Geometry check sheet. Reference: the model listing, model coordinates, mm. A direction names the side the tool comes from. Coordinates: 2 decimals unless noted, no trailing zeros. Loops run counter-clockwise (first coordinate to the right, second up) from the corner with the lowest first, then second, coordinate; pieces in that order, holes last.
Autodesk Inventor part; units mm, degrees
ref_plane "YZ Plane" through (0, 0, 0) normal (1, 0, 0) x (0, 1, 0)
ref_plane "XZ Plane" through (0, 0, 0) normal (0, 1, 0) x (-1, 0, 0)
ref_plane "XY Plane" through (0, 0, 0) normal (0, 0, 1) x (1, 0, 0)
sketch "Sketch1" plane through (0, 0, 0) normal (0, 1, 0) x (-1, 0, 0)
  line L0 (0, 0) -> (60, 0)
  line L1 (60, 0) -> (60, -140)
  line L2 (60, -140) -> (0, -140)
  line L3 (0, -140) -> (0, 0)
  line L4 (30, -20.8594) -> (30, -183.1932) construction
  line L5 (42.5, -21.7206) -> (42.5, -191.0157) construction
  line L6 (17.5, -21.7206) -> (17.5, -184.1979) construction
  circle A0 centre (42.5, -21) radius 1.5
  circle A1 centre (42.5, -41) radius 1.5
  circle A2 centre (42.5, -99) radius 1.5
  circle A3 centre (42.5, -119) radius 1.5
  circle A4 centre (17.5, -99) radius 1.5
  circle A5 centre (17.5, -119) radius 1.5
  circle A6 centre (17.5, -41) radius 1.5
  circle A7 centre (17.5, -21) radius 1.5
  dimension "d0" = 140
  dimension "d1" = 60
  dimension "d2" = 30
  dimension "d3" = 12.5
  dimension "d4" = 12.5
  dimension "d5" = 3
  dimension "d6" = 3
  dimension "d7" = 3
  dimension "d8" = 3
  dimension "d9" = 3
  dimension "d10" = 3
  dimension "d11" = 3
  dimension "d12" = 3
  dimension "d13" = 20
  dimension "d14" = 20
  dimension "d15" = 20
  dimension "d16" = 20
  dimension "d17" = 21
  dimension "d18" = 21
  dimension "d19" = 21
  dimension "d20" = 21
extrude "Extrusion1" add sketch "Sketch1" along normal blind 5
sketch "Sketch2" plane through (0, 0, 0) normal (0, -1, 0) x (1, 0, 0)
  circle A0 centre (-52.5, -120) radius 2.5
  circle A1 centre (-52.5, -20) radius 2.5
  circle A2 centre (-7.5, -120) radius 2.5
  circle A3 centre (-7.5, -20) radius 2.5
  line L0 (-60, -140) -> (-60, 0)
  line L1 (0, -140) -> (-60, -140)
  line L2 (-60, 0) -> (0, 0)
  line L3 (0, 0) -> (0, -140)
  dimension "d23" = 5
  dimension "d24" = 5
  dimension "d25" = 5
  dimension "d26" = 5
  dimension "d27" = 7.5
  dimension "d28" = 20
  dimension "d29" = 7.5
  dimension "d30" = 20
  dimension "d31" = 20
  dimension "d32" = 7.5
  dimension "d33" = 20
  dimension "d34" = 7.5
extrude "Extrusion2" cut sketch "Sketch2" against normal blind 10 contours A0 | A1 | A2 | A3
sketch "Sketch3" plane through (0, 0, 0) normal (0, -1, 0) x (1, 0, 0)
  line L0 (-68.3542, -70) -> (15.9682, -70) construction
  line L1 (0, -140) -> (-60, -140)
  line L2 (-35, -136) -> (-25, -136)
  line L3 (-25, -136) -> (-25, -131)
  line L4 (-25, -131) -> (-35, -131)
  line L5 (-35, -131) -> (-35, -136)
  line L6 (-60, -140) -> (-60, 0)
  line L7 (-35, -4) -> (-25, -4)
  line L8 (-25, -4) -> (-25, -9)
  line L9 (-25, -9) -> (-35, -9)
  line L10 (-35, -9) -> (-35, -4)
  point P0 (0, 0)
  dimension "d40" = 70
  dimension "d41" = 10
  dimension "d42" = 25
  dimension "d43" = 4
  dimension "d44" = 5
extrude "Extrusion3" cut sketch "Sketch3" against normal blind 10
fillet "Fillet2" radius 5 4 edges at (0, 2.5, -140) (-60, 2.5, -140) (-60, 2.5, 0) (0, 2.5, 0)
sketch "Sketch4" plane through (0, 5, 0) normal (0, 1, 0) x (1, 0, 0)
  circle A0 centre (-10, 65.5) radius 1.5
  circle A1 centre (-30, 65.5) radius 1.5
  circle A2 centre (-50, 65.5) radius 1.5
  line L0 (3.8133, 65.5) -> (-51.9818, 65.5) construction
  line L1 (-55, 0) -> (-5, 0)
  line L2 (0, 5) -> (0, 135)
  point P0 (0, 0)
  dimension "d49" = 3
  dimension "d50" = 3
  dimension "d51" = 3
  dimension "d52" = 65.5
  dimension "d53" = 10
  dimension "d54" = 30
  dimension "d55" = 50
extrude "Extrusion4" cut sketch "Sketch4" against normal blind 10
fillet "Fillet3" radius 2 8 edges at (-25, 2.5, -131) (-25, 2.5, -136) (-35, 2.5, -136) (-35, 2.5, -131) (-25, 2.5, -9) (-25, 2.5, -4) (-35, 2.5, -4) (-35, 2.5, -9)
equation "\"d2\" = 0.5 * d1"
equation "\"d4\" = d3"
equation "\"d6\" = d5"
equation "\"d7\" = d5"
equation "\"d8\" = d5"
equation "\"d9\" = d5"
equation "\"d10\" = d5"
equation "\"d11\" = d5"
equation "\"d12\" = d5"
equation "\"d14\" = d13"
equation "\"d15\" = d13"
equation "\"d16\" = d13"
equation "\"d18\" = d17"
equation "\"d19\" = d17"
equation "\"d20\" = d17"
equation "\"d29\" = d27"
equation "\"d30\" = d28"
equation "\"d31\" = d28"
equation "\"d32\" = d27"
equation "\"d33\" = d28"
equation "\"d34\" = d27"
properties part number "Y-Axis_back_plate_bottom"
1) Material ranges on probe 1 along X at (y, z) = (3.55, -65.5); probe 2 along X at (y, z) = (3.3, -99); probe 3 along Z at (x, y) = (-17.5, 1.2), recorded low to high.
Data:
probe 1: x = -60 to -51.5, -48.5 to -31.5, -28.5 to -11.5, -8.5 to 0
probe 2: x = -60 to -44, -41 to -19, -16 to 0
probe 3: z = -140 to -120.5, -117.5 to -100.5, -97.5 to -42.5, -39.5 to -22.5, -19.5 to 0
2) Section check B-B on y = 3.15. Count the separate pieces of the cut face and the enclosed holes in it, and give its area (3 significant figures).
Data:
separate pieces: 1
enclosed holes: 17
area: 8,130 mm2
3) Access from +Z, -Z, +X, -X, +Y, -Y to the whole of each face (thin tool, end or side, straight path). Record for faces 1 (the flat face through (-30, 2, -9)), 2 (the cylindrical face through (-1, 3, -138)).
Data:
face 1: +Y, -Y
face 2: -Z, +X, +Y, -Y
4) Mould release check, pull along Z, two halves, no side actions. Record for faces 3 (the cylindrical face through (-58, 3, -139)), 4 (the flat face through (-30, 2, -131)), 5 (the flat face through (-30, 0, -69)): +Z half, -Z half, draft (parallel to the pull), parting line (faces both ways), or undercut.
Data:
face 3: -Z half
face 4: undercut
face 5: draft
5) Section check A-A on z = -99. Record the cut outline in (x, y).
Data:
outline: (-60, 0) - (-44, 0) - (-44, 5) - (-60, 5) - close; (-41, 0) - (-19, 0) - (-19, 5) - (-41, 5) - close; (-16, 0) - (0, 0) - (0, 5) - (-16, 5) - close
